```python
from build123d import *

# Parameters (mm, degrees)
F1_DEPTH  = 25
F3_W      = 44.3
F3_H      = 19
F4_DEPTH  = 20
F5_W      = 10
F5_H      = 44.3
F6_DEPTH  = 25
F7_W      = 44.3
F7_H      = 19
F8_DEPTH  = 20
F9_W      = 10
F9_H      = 44.3
F10_DEPTH = 25
F11_W     = 44.3
F11_H     = 3.8
F12_DEPTH = 20
F13_W     = 44.3
F13_H     = 3.8
F14_DEPTH = 20
F16_DEPTH = 63
F2_W      = 40
F2_H      = 150.6
F17_DEPTH = 4
F19_DEPTH = 6.2
F20_W     = 6.3
F20_H     = 2.2
F21_DEPTH = 25


with BuildPart() as f1:
    # F0 (on Top) → F1 (new body)
    with BuildSketch(Plane.XY):
        Polygon((40.029135, -69.956624), (40.029135, 80.643376), (20.029135, 80.643376), (10.029135, 80.643376), (10.029135, 36.343376), (30.029135, 36.343376), (30.029135, -25.656624), (10.029135, -25.656624), (10.029135, -69.956624), (20.029135, -69.956624), align=None)
    extrude(amount=F1_DEPTH)

    # F3 (on face) → F4 (cut)
    with BuildSketch(Plane(origin=(10.029135, 0, 0), x_dir=(0, -1, 0), z_dir=(-1, 0, 0))):
        with Locations((-58.493376, 13.3)):
            Rectangle(F3_W, F3_H)
    extrude(amount=-F4_DEPTH, mode=Mode.SUBTRACT)

    # F5 (on face) → F6 (cut)
    with BuildSketch(Plane.XY.offset(25)):
        with Locations((15.029135, 58.493376)):
            Rectangle(F5_W, F5_H)
    extrude(amount=-F6_DEPTH, mode=Mode.SUBTRACT)

    # F7 (on face) → F8 (cut)
    with BuildSketch(Plane(origin=(10.029135, 0, 0), x_dir=(0, -1, 0), z_dir=(-1, 0, 0))):
        with Locations((47.806624, 13.3)):
            Rectangle(F7_W, F7_H)
    extrude(amount=-F8_DEPTH, mode=Mode.SUBTRACT)

    # F9 (on face) → F10 (cut)
    with BuildSketch(Plane.XY.offset(25)):
        with Locations((15.029135, -47.806624)):
            Rectangle(F9_W, F9_H)
    extrude(amount=-F10_DEPTH, mode=Mode.SUBTRACT)

    # F11 (on face) → F12 (join)
    with BuildSketch(Plane(origin=(20.029135, 0, 0), x_dir=(0, -1, 0), z_dir=(-1, 0, 0))):
        with Locations((-58.493376, 1.9)):
            Rectangle(F11_W, F11_H)
    extrude(amount=F12_DEPTH)

    # F13 (on face) → F14 (join)
    with BuildSketch(Plane(origin=(20.029135, 0, 0), x_dir=(0, -1, 0), z_dir=(-1, 0, 0))):
        with Locations((47.806624, 1.9)):
            Rectangle(F13_W, F13_H)
    extrude(amount=F14_DEPTH)

    # F15 (on face) → F16 (join)
    with BuildSketch(Plane(origin=(0, -25.656624, 0), x_dir=(-1, 0, 0), z_dir=(0, 1, 0))):
        Polygon((-0.029135, 3.8), (-30.029135, 3.8), (-30.029135, 0), (0, 0), align=None)
    extrude(amount=F16_DEPTH)

    # F2 (on face) → F17 (join)
    with BuildSketch(Plane(origin=(0, 0, 0), x_dir=(1, 0, 0), z_dir=(0, 0, -1))):
        with Locations((20.029135, -5.343376)):
            Rectangle(F2_W, F2_H)
    extrude(amount=F17_DEPTH)

    # F18 (on face) → F19 (cut)
    with BuildSketch(Plane(origin=(0, 0, -4), x_dir=(1, 0, 0), z_dir=(0, 0, -1))):
        Polygon((0.029135, -2.193376), (0.029135, -8.493376), (17.059135, -8.493376), (17.059135, -11.343376), (22.059135, -11.343376), (22.059135, 0.656624), (17.059135, 0.656624), (17.059135, -2.193376), align=None)
    extrude(amount=-F19_DEPTH, mode=Mode.SUBTRACT)

    # F20 (on face) → F21 (cut)
    with BuildSketch(Plane.YZ.offset(0.029135)):
        with Locations((5.343376, 1.1)):
            Rectangle(F20_W, F20_H)
    extrude(amount=-F21_DEPTH, mode=Mode.SUBTRACT)


solid = f1.part
```
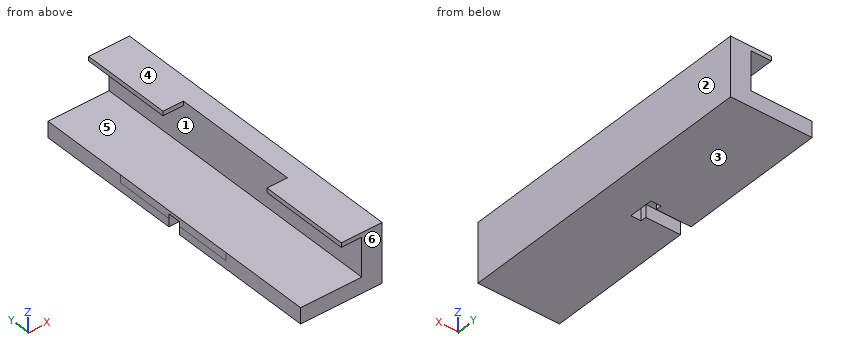
Source: CAD feature listing. Evaluate the final solid. Frame: model axes, mm. Face numbers are marked on the shaded views. A direction names the side the tool comes from. Coordinates: 2 decimals unless noted, no trailing zeros. Loops run counter-clockwise (first coordinate to the right, second up) from the corner with the lowest first, then second, coordinate; pieces in that order, holes last. Notation, with made-up numbers: (60.25, 6) -> (89.25, 6) arc R24 cw to (89.25, 45) -> close; hole circle Ø2 at (8.25, 79.25). An arc over 180 degrees is marked (long way). One line per item, written item: value. Start each with the question number.
Q1. Section query C-C, the plane x = 15.5. Return the cut outline in (y, z).
Q2. Mould query, pull axis Z, two halves, no side actions, for the marked faces 1, 2, 3 and 4. Classes: pulls with the +Z half, pulls with the -Z half, needs draft (parallel to the pull), parting line crosses it, or undercut.
Q3. Line query: line 1 along Z through (x, y) = (27, -37); line 2 along Y through (x, z) = (11.5, 0); line 3 along Y through (x, z) = (27.5, 23.25). Output: solid intervals per line, ascending.
Q4. Section query B-B, the plane y = 41. Return the cut outline in (x, z).
Q5. Section query A-A, the plane x = 25. Return the cut outline in (y, z).
Q6. Set-up query: the marked faces 5 and 6. Return all of +Z, -Z, +X, -X, +Y, -Y with unobstructed straight access to the full face (end or side cutting, diameter ignored); none if empty.
Q7. Section query D-D, the plane z = 13.5. Return the cut outline in (x, y).
Q8. Contact query for flat-ended pins moving along their axis: P1, Ø5, axis at y = -54, z = 16.5, coming from the -X side; P2, Ø24, axis at x = 17, y = -4, coming from the +Z side; P3, Ø17, axis at y = 26, z = 10, coming from the -X side; P4, Ø2, axis at x = 11.5, z = 5, coming from the +Y side. Output: stop coordinate, or through.
Results:
1. outline: (-69.96, -4) -> (2.19, -4) -> (2.19, 2.2) -> (8.49, 2.2) -> (8.49, -4) -> (80.64, -4) -> (80.64, 3.8) -> (-69.96, 3.8) -> close
2. face 1: undercut
2. face 2: needs draft
2. face 3: pulls with the -Z half
2. face 4: pulls with the +Z half
3. line 1: -4 to 3.8, 22.8 to 25
3. line 2: -69.96 to 2.19, 8.49 to 80.64
3. line 3: -69.96 to -25.66, 36.34 to 80.64
4. outline: (0.03, -4) -> (40.03, -4) -> (40.03, 25) -> (20.03, 25) -> (20.03, 22.8) -> (30.03, 22.8) -> (30.03, 3.8) -> (0.03, 3.8) -> close
5. outline: (-69.96, -4) -> (80.64, -4) -> (80.64, 3.8) -> (-69.96, 3.8) -> close; (-69.96, 22.8) -> (-25.66, 22.8) -> (-25.66, 25) -> (-69.96, 25) -> close; (36.34, 22.8) -> (80.64, 22.8) -> (80.64, 25) -> (36.34, 25) -> close
6. face 5: -X, +Y, -Y
6. face 6: +Z, -Z, +X, -X, -Y
7. outline: (30.03, -69.96) -> (40.03, -69.96) -> (40.03, 80.64) -> (30.03, 80.64) -> close
8. P1: x = 30.03
8. P2: z = 3.8
8. P3: x = 0.01
8. P4: through
